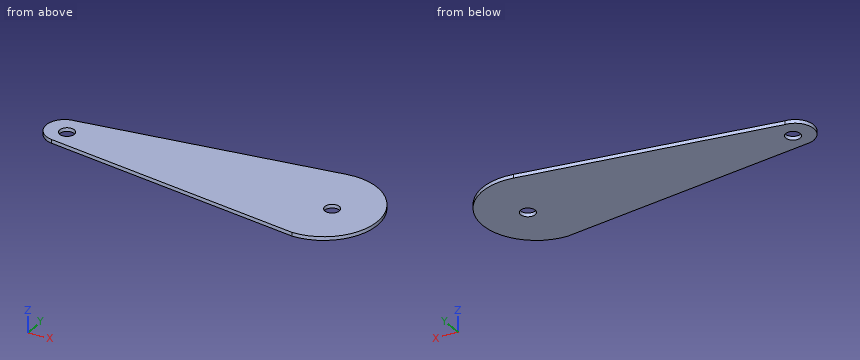
```python
from build123d import *

# Parameters (mm, degrees)
BOSS_EXTRUDE1_DEPTH = 1
SKETCH2_R           = 2.000000064
CUT_EXTRUDE1_DEPTH  = 2.54
SCALE1_SCALE        = 1.3


with BuildPart() as part:
    # Sketch1 → Boss-Extrude1 (new body)
    with BuildSketch(Plane.XY):
        with BuildLine():
            Line((-69.316067153, 3.878962407), (-2.316488686, 14.547627491))
            ThreePointArc((-2.316488686, 14.547627491), (14.685052241, 1.161389736), (-0.000951264, -14.730905761))
            Line((-0.000951264, -14.730905761), (-69.753484787, -6.240756815))
            ThreePointArc((-69.753484787, -6.240756815), (-74.214947759, -0.978600121), (-69.316067153, 3.878962407))
        make_face()
    extrude(amount=BOSS_EXTRUDE1_DEPTH)

    # Sketch2 → Cut-Extrude1 (cut)
    with BuildSketch(Plane(origin=(0, 0, 0), x_dir=(-1, 0, 0), z_dir=(0, 0, -1))):
        with Locations((-2.636515213, -0.692372509)):
            Circle(SKETCH2_R)
        with Locations((68.361932579, -1.498185023)):
            Circle(SKETCH2_R)
    extrude(amount=-CUT_EXTRUDE1_DEPTH, mode=Mode.SUBTRACT)


with BuildPart() as part_1:
    # Scale1: scaled about (-22.971903001, -0.371312975, 0.5)
    add(part.part.scale(SCALE1_SCALE).moved(Location((6.8915709, 0.111393893, -0.15))))


solid = part_1.part
```
Geometry check sheet. Reference: the model listing, model coordinates, mm. Coordinates: 2 decimals unless noted, no trailing zeros. Write each loop counter-clockwise with the first axis right and the second up, starting at its lowest first coordinate (ties: lowest second). Pieces come first, ordered by that corner, then holes. Notation, with made-up numbers: M 24,-18 L 71,-18 A19 cw 71,15 Z; hole C 65.25,25 d1. An arc over 180 degrees is marked long. Answer as a JSON object with one key per item and string values.
1. Section check D-D, the plane x = 14.5. Enter the section's corners in (y, z), plus the area to 3 significant figures.
Answers below:
{"outline": "M -17.46,-0.15 L 17.69,-0.15 L 17.69,1.15 L -17.46,1.15 Z", "area": "45.7 mm²"}
2. Section check B-B, the plane z = 0.45. Enter the section's corners in (x, y), plus the area to 3 significant figures.
Answers below:
{"outline": "M -83.79,-8 L 6.89,-19.04 A19.15 ccw long 3.88,19.02 L -83.22,5.15 A6.6 ccw Z; hole C -81.98,-1.84 d5.2; hole C 10.32,-0.79 d5.2", "area": "2,930 mm²"}
3. Scan lines: L1, parallel to X at y = -3, z = 0.2; L2, parallel to X at y = -2, z = 1 (3 decimals); L3, parallel to Y at x = 7, z = 0.85. Record each from-to range of solid material in increasing order.
Answers below:
{"L1": "x = -89.41 to -84.3, -79.65 to 8.95, 11.69 to 25.79", "L2": "x = -89.571 to -84.574, -79.384 to 8.018, 12.62 to 25.925", "L3": "y = -19.04 to 19.26"}
4. Section check A-A, the plane x = -81. Enter the section's corners in (y, z).
Answers below:
{"outline": "M -8.34,-0.15 L -4.24,-0.15 L -4.24,1.15 L -8.34,1.15 Z; M 0.57,-0.15 L 5.51,-0.15 L 5.51,1.15 L 0.57,1.15 Z"}
5. Section check C-C, the plane x = -22.5. Enter the section's corners in (y, z), plus the area to 3 significant figures.
Answers below:
{"outline": "M -15.46,-0.15 L 14.82,-0.15 L 14.82,1.15 L -15.46,1.15 Z", "area": "39.4 mm²"}
